Design review of the part built by this model. Coordinates are the model's own, in mm. A direction names the side the tool comes from. Coordinates: 2 decimals unless noted, no trailing zeros. Loops run counter-clockwise (first coordinate to the right, second up) from the corner with the lowest first, then second, coordinate; pieces in that order, holes last.
from build123d import *

# Parameters (mm, degrees)
BOSS_EXTRUDE12_DEPTH = 3
SKETCH1_16_W         = 18.27
SKETCH1_16_H         = 13.8
SKETCH1_16_W_2       = 18.57
SKETCH1_16_W_3       = 32.07
BOSS_EXTRUDE13_DEPTH = 10
SKETCH1_17_W         = 13.8
SKETCH1_17_H         = 13.8
BOSS_EXTRUDE14_DEPTH = 6.5
FILLET1_R            = 1


with BuildPart() as part:
    # Sketch1 → Boss-Extrude12 (new body)
    with BuildSketch(Plane(origin=(0, 0, 0), x_dir=(1, 0, 0), z_dir=(0, 1, 0))):
        with BuildLine():
            ThreePointArc((90.24192642, 0), (100, 0), (100, 9.75807358))
            Line((100, 9.75807358), (91.252103749, 18.505969831))
            ThreePointArc((91.252103749, 18.505969831), (13.301158056, 86.698841944), (81.494030169, 8.747896251))
            Line((81.494030169, 8.747896251), (90.24192642, 0))
        make_face()
    extrude(amount=BOSS_EXTRUDE12_DEPTH)

    # Sketch1_16 → Boss-Extrude13 (add)
    with BuildSketch(Plane(origin=(0, 0, 0), x_dir=(1, 0, 0), z_dir=(0, 1, 0))):
        with BuildLine():
            ThreePointArc((90.24192642, 0), (100, 0), (100, 9.75807358))
            Line((100, 9.75807358), (91.252103749, 18.505969831))
            ThreePointArc((91.252103749, 18.505969831), (13.301158056, 86.698841944), (81.494030169, 8.747896251))
            Line((81.494030169, 8.747896251), (90.24192642, 0))
        make_face()
        with BuildLine():
            Line((36.2, 56.9), (10.599619291, 56.9))
            ThreePointArc((10.599619291, 56.9), (11.37337625, 60.391532017), (12.455892606, 63.8))
            Line((12.455892606, 63.8), (43.1, 63.8))
            Line((43.1, 63.8), (43.1, 77.6))
            Line((43.1, 77.6), (21.047625313, 77.6))
            ThreePointArc((21.047625313, 77.6), (90, 50), (21.047625313, 22.4))
            Line((21.047625313, 22.4), (29.3, 22.4))
            Line((29.3, 22.4), (29.3, 36.2))
            Line((29.3, 36.2), (12.455892606, 36.2))
            ThreePointArc((12.455892606, 36.2), (11.37337625, 39.608467983), (10.599619291, 43.1))
            Line((10.599619291, 43.1), (36.2, 43.1))
            Line((36.2, 43.1), (36.2, 56.9))
        make_face(mode=Mode.SUBTRACT)
        with Locations((59.135, 70.7)):
            Rectangle(SKETCH1_16_W, SKETCH1_16_H)
        with Locations((73.085, 50)):
            Rectangle(SKETCH1_16_W_2, SKETCH1_16_H)
        with Locations((52.235, 29.3)):
            Rectangle(SKETCH1_16_W_3, SKETCH1_16_H)
    extrude(amount=BOSS_EXTRUDE13_DEPTH)

    # Sketch1_17 → Boss-Extrude14 (add)
    with BuildSketch(Plane(origin=(0, 0, 0), x_dir=(1, 0, 0), z_dir=(0, 1, 0))):
        with Locations((50, 50)):
            Rectangle(SKETCH1_17_W, SKETCH1_17_H)
    extrude(amount=BOSS_EXTRUDE14_DEPTH)

    # Fillet1
    fillet1_edges = [part.edges().sort_by_distance(p)[0] for p in [
        (43.1, 3, -50),
        (50, 3, -43.1),
        (56.9, 3, -50),
        (50, 3, -56.9),
        (50, 3, -70.7),
        (59.135, 3, -63.8),
        (68.27, 3, -70.7),
        (59.135, 3, -77.6),
        (36.2, 3, -29.3),
        (52.235, 3, -22.4),
        (68.27, 3, -29.3),
        (52.235, 3, -36.2),
        (63.8, 3, -50),
        (73.085, 3, -43.1),
        (82.37, 3, -50),
        (73.085, 3, -56.9),
        (23.399809646, 3, -43.1),
        (27.777946303, 3, -63.8),
        (25.173812657, 3, -22.4),
        (11.37337625, 3, -39.608467983),
        (36.2, 3, -50),
        (23.399809646, 3, -56.9),
        (11.37337625, 3, -60.391532017),
        (43.1, 3, -70.7),
        (32.073812657, 3, -77.6),
        (90, 3, -50),
        (29.3, 3, -29.3),
        (20.877946303, 3, -36.2),
    ]]
    fillet(fillet1_edges, radius=FILLET1_R)


solid = part.part
Q1. For line 1 (X direction, y = 7.6, z = -50); line 2 (X direction, y = 6.1, z = -50); line 3 (Z direction, x = 51.5, y = 5.25), list the stretches that pass through material, from the lowest coordinate up.
Q2. Clearance check with flat-ended pins moving along their axes: pin 1 Ø5 at (x, y) = (23, 6) entering from -Z; pin 2 Ø3 at (y, z) = (6.5, -74) entering from -X; pin 3 Ø1 at (y, z) = (4, -51.5) entering from -X. State where each tip first meets the part, or that it passes through.
Q3. Machinability: for faces 1 (the flat face through (68.27, 7, -71)), 2 (the flat face through (26, 10, -51)), which of the approach directions +Z, -Z, +X, -X, +Y, -Y give a long, thin tool a straight path to every point of the face, cutting with its end or side? Answer none if there is none.
Q4. Take a section at B-B, the plane z = -50. Write out the cut boundary in (x, y), then the cut area to 3 significant figures.
Q5. The part is to be moulded in two halves that separate along X. For faces 3 (the flat face through (25, 7, -22.4)), 4 (the flat face through (49, 0, -51)), say which applies: pulls with the +X half, pulls with the -X half, needs draft (parallel to the pull), parting line crosses it, or undercut.
Q6. Take a section at A-A, the plane y = 5.25. Give the number of separate pieces and of enclosed holes in the cut face, then the cut area to 3 significant figures.
Entries:
1. line 1: x = -1.9 to 36.2, 63.8 to 82.37, 90 to 101.9
1. line 2: x = -1.9 to 36.2, 43.1 to 56.9, 63.8 to 82.37, 90 to 101.9
1. line 3: z = -101.88 to -89.97, -77.6 to -63.8, -56.9 to -43.1, -36.2 to -22.4, -10.03 to 1.88
2. pin 1: stops at z = -95.75
2. pin 2: stops at x = 3.23
2. pin 3: stops at x = -1.89
3. face 1: +Y
3. face 2: +Z, -Z, +X, -X, +Y
4. outline: (-1.9, 0) - (101.9, 0) - (101.9, 10) - (90, 10) - (90, 4) arc R1 cw to (89, 3) - (83.37, 3) arc R1 cw to (82.37, 4) - (82.37, 10) - (63.8, 10) - (63.8, 4) arc R1 cw to (62.8, 3) - (57.9, 3) arc R1 cw to (56.9, 4) - (56.9, 6.5) - (43.1, 6.5) - (43.1, 4) arc R1 cw to (42.1, 3) - (37.2, 3) arc R1 cw to (36.2, 4) - (36.2, 10) - (-1.9, 10) - close
4. area: 841 mm2
5. face 3: undercut
5. face 4: needs draft
6. separate pieces: 5
6. enclosed holes: 1
6. area: 5,730 mm2
